Could you check a few things on this drawing? It's one solid part, dimensions in mm from its lowest x, y, z. A direction names the side the tool comes from. Coordinates: 2 decimals unless noted, no trailing zeros. Write each loop counter-clockwise with the first axis right and the second up, starting at its lowest first coordinate (ties: lowest second). Pieces come first, ordered by that corner, then holes. Notation, with made-up numbers: (64, 16.25) - (104, 16.25) arc R21 cw to (104, 34.25) - close; hole circle Ø1 at (-31, 6). An arc over 180 degrees is marked (long way). Answer as a JSON object with one key per item and string values. Group by question number.
1) If we section it at D-D (x = 11.5): Write out the boundary of the cut face in (y, z).
2) Will these pins go through, and if not, where does the flat tip stop? pin 1 Ø6 at (x, y) = (30.5, 6.5) entering from +Z; pin 2 Ø8.5 at (x, y) = (25, 20) entering from -Z; pin 3 Ø1.5 at (x, y) = (22.5, 29) entering from +Z.
3) On a 3-axis mill with a long thin cutter (end or side, diameter ignored), from which of +Z, -Z, +X, -X, +Y, -Y can I reach the whole of each face in a straight line? I mean the marked faces 1, 2 and 3. Say none if no direction works.
4) If we section it at C-C (y = 8.5): Write out the boundary of the cut face in (x, z).
5) If we section it at A-A (z = 10.16): Write out the boundary of the cut face in (x, y).
6) Please list where these lines run through material, in increasing order: line 1 along Z through (x, y) = (1, 19); line 2 along X through (y, z) = (22, 73.5); line 3 along Y through (x, z) = (1.25, 10.16).
7) If we section it at B-B (z = 82): Write out the boundary of the cut face in (x, y), plus the area to 3 significant figures.
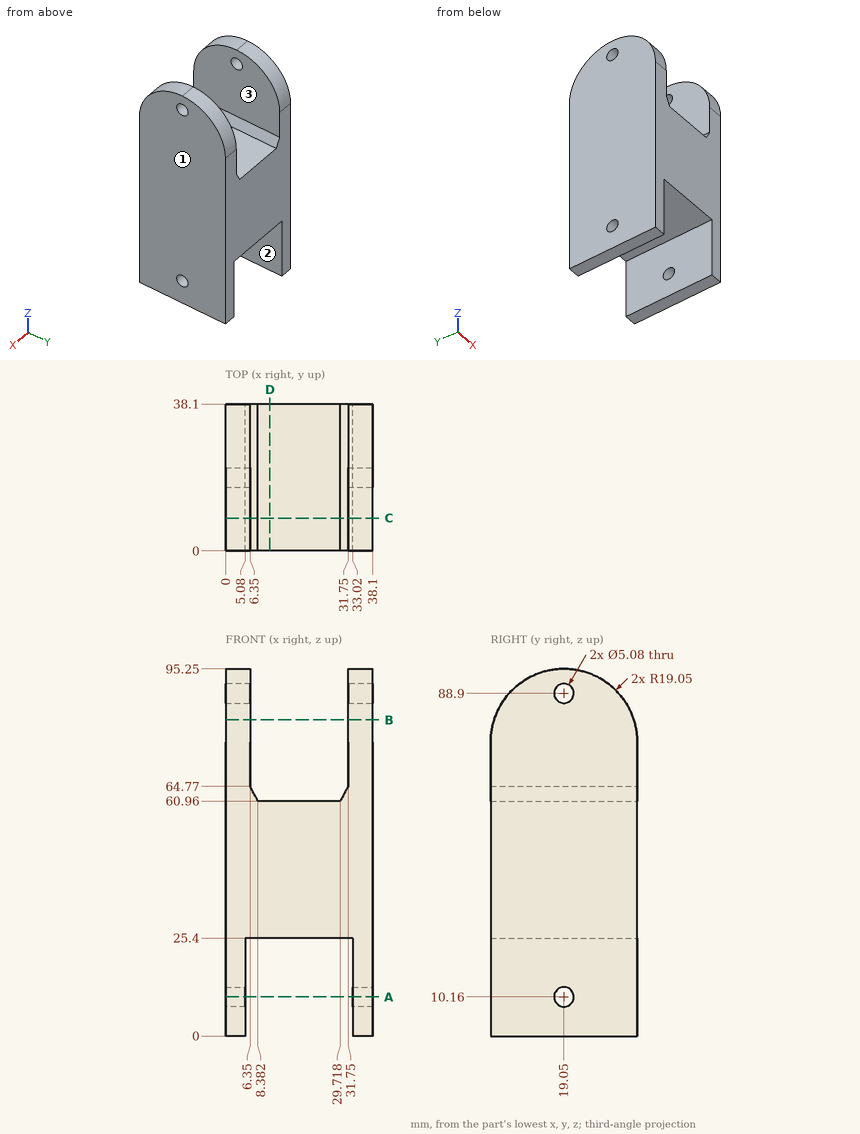
Here are the results:
{
 "1": {"outline": "(0, 25.4) - (38.1, 25.4) - (38.1, 60.96) - (0, 60.96) - close"},
 "2": {"pin 1": "stops at z = 92.52", "pin 2": "stops at z = 25.4", "pin 3": "stops at z = 60.96"},
 "3": {"face 1": "+Z, -Z, +X, +Y, -Y", "face 2": "-Z, +Y, -Y", "face 3": "+Z, +Y, -Y"},
 "4": {"outline": "(0, 0) - (5.08, 0) - (5.08, 25.4) - (33.02, 25.4) - (33.02, 0) - (38.1, 0) - (38.1, 92.06) - (31.75, 92.06) - (31.75, 64.77) - (29.72, 60.96) - (8.38, 60.96) - (6.35, 64.77) - (6.35, 92.06) - (0, 92.06) - close"},
 "5": {"outline": "(0, 0) - (5.08, 0) - (5.08, 16.51) - (0, 16.51) - close; (0, 21.59) - (5.08, 21.59) - (5.08, 38.1) - (0, 38.1) - close; (33.02, 0) - (38.1, 0) - (38.1, 16.51) - (33.02, 16.51) - close; (33.02, 21.59) - (38.1, 21.59) - (38.1, 38.1) - (33.02, 38.1) - close"},
 "6": {"line 1": "z = 0 to 7.62, 12.7 to 86.36, 91.44 to 95.25", "line 2": "x = 0 to 6.35, 31.75 to 38.1", "line 3": "y = 0 to 16.51, 21.59 to 38.1"},
 "7": {"outline": "(0, 0.9) - (6.35, 0.9) - (6.35, 37.2) - (0, 37.2) - close; (31.75, 0.9) - (38.1, 0.9) - (38.1, 37.2) - (31.75, 37.2) - close", "area": "461 mm²"}
}
